Autodesk Inventor part; units mm, degrees
ref_plane "YZ Plane" through (0, 0, 0) normal (1, 0, 0) x (0, 1, 0)
ref_plane "XZ Plane" through (0, 0, 0) normal (0, 1, 0) x (-1, 0, 0)
ref_plane "XY Plane" through (0, 0, 0) normal (0, 0, 1) x (1, 0, 0)
sketch "Sketch1" plane through (0, 0, 0) normal (0, 1, 0) x (-1, 0, 0)
  line L0 (21.5, 8.8) -> (-21.5, 8.8)
  line L1 (-21.5, 8.8) -> (-21.5, -8.8)
  line L2 (-21.5, -8.8) -> (21.5, -8.8)
  line L3 (21.5, -8.8) -> (21.5, 8.8)
  line L4 (21.5, 8.8) -> (-21.5, -8.8) construction
  line L5 (-21.5, 8.8) -> (21.5, -8.8) construction
  line L6 (20.5, 7.8) -> (-20.5, 7.8) construction
  line L7 (-20.5, 7.8) -> (-20.5, -7.8) construction
  line L8 (-20.5, -7.8) -> (20.5, -7.8) construction
  line L9 (20.5, -7.8) -> (20.5, 7.8) construction
  point P0 (0, 0)
  dimension "d0" = 43
  dimension "d1" = 17.6
  dimension "d2" = 1
extrude "Extrusion1" add sketch "Sketch1" against normal blind 1.5
hole "Hole1" at (-20.5, 0, 7.8) at (-20.5, 0, -7.8) at (20.5, 0, 7.8) at (20.5, 0, -7.8) direction (0, -1, 0) diameter 1 end through all
sketch "Sketch2" plane through (0, 0, 0) normal (0, 1, 0) x (1, 0, 0)
  line L0 (-21.5, 3.75) -> (-16.5, 3.75)
  line L1 (-16.5, 3.75) -> (-16.5, -3.75)
  line L2 (-16.5, -3.75) -> (-21.5, -3.75)
  line L3 (-21.5, -3.75) -> (-21.5, 3.75)
  line L4 (-21.5, 3.75) -> (-16.5, -3.75) construction
  line L5 (-16.5, 3.75) -> (-21.5, -3.75) construction
  line L6 (-21.5, 8.8) -> (-21.5, -8.8)
  point P0 (0, 0)
  point P1 (-19, 0)
  point P2 (-21.5, 0)
  dimension "d12" = 5
  dimension "d13" = 7.5
extrude "Extrusion2" add sketch "Sketch2" along normal blind 9
sketch "Sketch3" plane through (0, 0, 0) normal (0, 1, 0) x (1, 0, 0)
  point P0 (0, 0)
sketch "Sketch4" plane through (0, 0, 0) normal (0, 1, 0) x (1, 0, 0)
  line L0 (13.6557, 4) -> (22.6557, 4)
  line L1 (22.6557, 4) -> (22.6557, -4)
  line L2 (22.6557, -4) -> (13.6557, -4)
  line L3 (13.6557, -4) -> (13.6557, 4)
  line L4 (13.6557, 4) -> (22.6557, -4) construction
  line L5 (22.6557, 4) -> (13.6557, -4) construction
  point P0 (0, 0)
  point P1 (18.1557, 0)
  dimension "d16" = 9
  dimension "d17" = 8
extrude "Extrusion3" add sketch "Sketch4" along normal blind 4
sketch "Sketch5" plane through (0, -1.5, 0) normal (0, -1, 0) x (1, 0, 0)
  circle A0 centre (20.5, 7.8) radius 0.5 construction
  circle A1 centre (-20.5, 7.8) radius 0.5 construction
  circle A2 centre (-20.5, -7.8) radius 0.5 construction
  circle A3 centre (20.5, -7.8) radius 0.5 construction
  line L0 (21.5, -8.8) -> (21.5, 8.8) construction
  line L1 (21.5, 8.8) -> (-21.5, 8.8) construction
  line L2 (-21.5, 8.8) -> (-21.5, -8.8) construction
  line L3 (-21.5, -8.8) -> (21.5, -8.8) construction
  line L4 (-20, 8.3) -> (20, 8.3)
  line L5 (20, 8.3) -> (20, 7.3)
  line L6 (20, 7.3) -> (-20, 7.3)
  line L7 (-20, 7.3) -> (-20, 8.3)
  line L8 (20, -8.3) -> (-20, -8.3)
  line L9 (-20, -8.3) -> (-20, -7.3)
  line L10 (-20, -7.3) -> (20, -7.3)
  line L11 (20, -7.3) -> (20, -8.3)
  point P0 (0, 0)
extrude "Extrusion4" add sketch "Sketch5" along normal blind 9
properties part number "nano_footprint"
Here's how the part is built. I have some questions about the finished solid (model axes, mm). A direction names the side the tool comes from. Give positions to 0.01 mm unless a question says otherwise; leave off trailing zeros. Order: outer loops, then holes, each group sorted by start corner. A loop starts at its lowest first (then second) coordinate and runs counter-clockwise, first axis right, second up. Notation, with made-up numbers: (58.25, 55.5) - (65.25, 55.5) arc R11 ccw to (65.25, 71.5) - close; hole circle Ø8 at (45.25, 70). An arc over 180 degrees is marked (long way). Answer as a JSON object with one key per item and string values. Group by question number.
Item 1: If we section it at C-C on z = 1.75: Please give me the cut outline in (x, y).
Item 2: Which directions (+Z, -Z, +X, -X, +Y, -Y) give clear straight access to the entire face, cutting with the end or side of a thin tool? Please do faces 5 (the flat face through (0, -6, 7.3)), 6 (the flat face through (0, -6, -8.3)), 7 (the flat face through (-19, 4, 3.75)), 8 (the flat face through (0, -6, 8.3)), 9 (the flat face through (21.5, -1, 0)).
Item 3: If we section it at D-D on x = 5.5: Please give me the cut outline in (y, z).
Item 4: If we mould it in two halves opening along X, with no side actions, what happens to faces 1 (the flat face through (20, -6, 8)), 2 (the flat face through (-21.5, 3, 0)), 3 (the flat face through (-16.5, 4, 0)), 4 (the flat face through (0, -1.5, 0))? For each: pulls with the +X half, pulls with the -X half, needs draft (parallel to the pull), parting line crosses it, or undercut.
Item 5: If we section it at B-B on x = -20.5: Please give me the cut outline in (y, z), and give its area (3 significant figures).
Item 6: Please list where these lines run through material, in increasing order: probe 1 along Z at (x, y) = (20.5, -0.5); probe 2 along X at (y, z) = (-0.5, 7.8); probe 3 along X at (y, z) = (2.25, -2).
Item 7: For P1, Ø7, axis at x = -1.5, y = -7, coming from the +Z side; P2, Ø2, axis at x = 12, y = 5.5, coming from the -Z side (3 decimals); P3, Ø1.1, axis at y = -7.5, z = 7.5, coming from the +X side; P4, Ø4, axis at x = -19.5, y = 3, coming from the -Z side, each with a flat end and sliding along its axis, tell me the tip position at first contact or that it passes through.
Item 8: If we section it at A-A on y = 1: Please give me the cut outline in (x, z).
Result set:
{
 "1": {"outline": "(-21.5, -1.5) - (21.5, -1.5) - (21.5, 0) - (22.66, 0) - (22.66, 4) - (13.66, 4) - (13.66, 0) - (-16.5, 0) - (-16.5, 9) - (-21.5, 9) - close"},
 "2": {"face 5": "+X, -X, -Y", "face 6": "-Z, +X, -X, -Y", "face 7": "+Z, -X, +Y", "face 8": "+Z, +X, -X, -Y", "face 9": "+Z, -Z, +X, -Y"},
 "3": {"outline": "(-10.5, -8.3) - (-1.5, -8.3) - (-1.5, -8.8) - (0, -8.8) - (0, 8.8) - (-1.5, 8.8) - (-1.5, 8.3) - (-10.5, 8.3) - (-10.5, 7.3) - (-1.5, 7.3) - (-1.5, -7.3) - (-10.5, -7.3) - close"},
 "4": {"face 1": "pulls with the +X half", "face 2": "pulls with the -X half", "face 3": "undercut", "face 4": "needs draft"},
 "5": {"outline": "(-1.5, -8.8) - (0, -8.8) - (0, -8.3) - (-1.5, -8.3) - close; (-1.5, -7.3) - (0, -7.3) - (0, -3.75) - (9, -3.75) - (9, 3.75) - (0, 3.75) - (0, 7.3) - (-1.5, 7.3) - close; (-1.5, 8.3) - (0, 8.3) - (0, 8.8) - (-1.5, 8.8) - close", "area": "90.9 mm²"},
 "6": {"probe 1": "-8.8 to -8.3, -7.3 to 7.3, 8.3 to 8.8", "probe 2": "-21.5 to -21, -20 to 20, 21 to 21.5", "probe 3": "-21.5 to -16.5, 13.66 to 22.66"},
 "7": {"P1": "z = 8.3", "P2": "through", "P3": "x = 20", "P4": "z = -3.75"},
 "8": {"outline": "(-21.5, -3.75) - (-16.5, -3.75) - (-16.5, 3.75) - (-21.5, 3.75) - close; (13.66, -4) - (22.66, -4) - (22.66, 4) - (13.66, 4) - close"}
}
